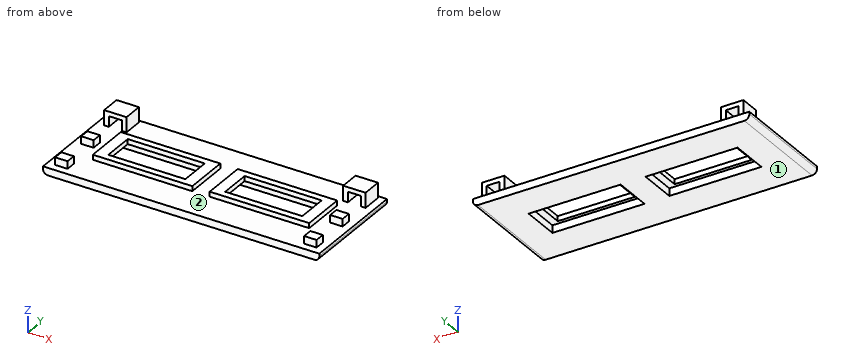
```python
from build123d import *

# Parameters (mm, degrees)
SKETCH1_W           = 111.1
SKETCH1_H           = 51.3
BOSS_EXTRUDE1_DEPTH = 3
SKETCH2_W           = 111.1
SKETCH2_H           = 51.3
SKETCH2_W_2         = 105.3
SKETCH2_H_2         = 45.3
BOSS_EXTRUDE2_DEPTH = 40.5
SKETCH10_W          = 126.244554882
SKETCH10_H          = 68.697179438
CUT_EXTRUDE2_DEPTH  = 53
SKETCH11_W          = 5
SKETCH11_H          = 4
BOSS_EXTRUDE7_DEPTH = 3
SKETCH12_W          = 9
SKETCH12_H          = 8
BOSS_EXTRUDE8_DEPTH = 6
SKETCH13_W          = 5.2
SKETCH13_H          = 4.2
CUT_EXTRUDE3_DEPTH  = 12
FILLET2_R           = 2
SKETCH5_W           = 37
SKETCH5_H           = 15.3
CUT_EXTRUDE5_DEPTH  = 3
SKETCH15_W          = 40
SKETCH15_H          = 18
SKETCH15_W_2        = 31
SKETCH15_H_2        = 12.5
BOSS_EXTRUDE9_DEPTH = 2


with BuildPart() as part:
    # Sketch1 → Boss-Extrude1 (new body)
    with BuildSketch(Plane(origin=(0, 0, 0), x_dir=(1, 0, 0), z_dir=(0, 1, 0))):
        Rectangle(SKETCH1_W, SKETCH1_H)
    extrude(amount=BOSS_EXTRUDE1_DEPTH)

    # Sketch2 → Boss-Extrude2 (add)
    with BuildSketch(Plane(origin=(0, 3, 0), x_dir=(1, 0, 0), z_dir=(0, 1, 0))):
        Rectangle(SKETCH2_W, SKETCH2_H)
        Rectangle(SKETCH2_W_2, SKETCH2_H_2, mode=Mode.SUBTRACT)
    extrude(amount=BOSS_EXTRUDE2_DEPTH)

    # Sketch10 → Cut-Extrude2 (cut)
    with BuildSketch(Plane.XY.offset(-22.65)):
        with Locations((0, 21.75)):
            Rectangle(SKETCH10_W, SKETCH10_H)
    extrude(amount=CUT_EXTRUDE2_DEPTH, mode=Mode.SUBTRACT)

    # Sketch11 → Boss-Extrude7 (add)
    with BuildSketch(Plane.XY.offset(-22.65)):
        with Locations((-50.05, 21.75)):
            Rectangle(SKETCH11_W, SKETCH11_H)
        with Locations((-50.05, 5)):
            Rectangle(SKETCH11_W, SKETCH11_H)
        with Locations((50.05, 5)):
            Rectangle(SKETCH11_W, SKETCH11_H)
        with Locations((50.05, 21.75)):
            Rectangle(SKETCH11_W, SKETCH11_H)
    extrude(amount=BOSS_EXTRUDE7_DEPTH)

    # Sketch12 → Boss-Extrude8 (add)
    with BuildSketch(Plane.XY.offset(-22.65)):
        with Locations((-48.05, 38.5)):
            Rectangle(SKETCH12_W, SKETCH12_H)
        with Locations((48.05, 38.5)):
            Rectangle(SKETCH12_W, SKETCH12_H)
    extrude(amount=BOSS_EXTRUDE8_DEPTH)

    # Sketch13 → Cut-Extrude3 (cut)
    with BuildSketch(Plane(origin=(0, 42.5, 0), x_dir=(1, 0, 0), z_dir=(0, 1, 0))):
        with Locations((-48.05, 20.55)):
            Rectangle(SKETCH13_W, SKETCH13_H)
        with Locations((48.05, 20.55)):
            Rectangle(SKETCH13_W, SKETCH13_H)
    extrude(amount=-CUT_EXTRUDE3_DEPTH, mode=Mode.SUBTRACT)

    # Fillet2
    fillet2_edges = [part.edges().sort_by_distance(p)[0] for p in [
        (-55.55, 21.75, -25.65),
        (55.55, 21.75, -25.65),
    ]]
    fillet(fillet2_edges, radius=FILLET2_R)

    # Sketch5 → Cut-Extrude5 (cut)
    with BuildSketch(Plane(origin=(0, 0, -25.65), x_dir=(-1, 0, 0), z_dir=(0, 0, -1))):
        with Locations((23.5, 21.75)):
            Rectangle(SKETCH5_W, SKETCH5_H)
        with Locations((-23.5, 21.75)):
            Rectangle(SKETCH5_W, SKETCH5_H)
    extrude(amount=-CUT_EXTRUDE5_DEPTH, mode=Mode.SUBTRACT)

    # Sketch15 → Boss-Extrude9 (add)
    # profile 1 of 2: a face of its own
    with BuildSketch(Plane.XY.offset(-22.65)):
        with Locations((23.5, 21.75)):
            Rectangle(SKETCH15_W, SKETCH15_H)
        with Locations((23.5, 21.75)):
            Rectangle(SKETCH15_W_2, SKETCH15_H_2, mode=Mode.SUBTRACT)
    # profile 2 of 2: a face of its own
    with BuildSketch(Plane.XY.offset(-22.65)):
        with Locations((-23.5, 21.75)):
            Rectangle(SKETCH15_W, SKETCH15_H)
        with Locations((-23.5, 21.75)):
            Rectangle(SKETCH15_W_2, SKETCH15_H_2, mode=Mode.SUBTRACT)
    extrude(amount=BOSS_EXTRUDE9_DEPTH)


solid = part.part
```
For this review, take the finished solid that the model builds, in its own axes (mm). Face numbers are marked on the shaded views. Coordinates: 2 decimals unless noted, no trailing zeros. Order: outer loops, then holes, each group sorted by start corner. A loop starts at its lowest first (then second) coordinate and runs counter-clockwise, first axis right, second up. Notation, with made-up numbers: (85, 27) - (93, 27) arc R26 cw to (93, 65) - close; hole circle Ø11 at (53.25, -39.75). An arc over 180 degrees is marked (long way). Answer as a JSON object with one key per item and string values. Group by question number.
1. The part is to be moulded in two halves that separate along X. For the marked faces 1 and 2, say which applies: pulls with the +X half, pulls with the -X half, needs draft (parallel to the pull), parting line crosses it, or undercut.
2. We need section A-A on x = -46.5. State the section outline as (y, z) points, then the cut area to 3 significant figures.
3. We need section B-B on y = 18. Give the number of separate pieces and of enclosed holes in the cut face, then the cut area to 3 significant figures.
4. We need section C-C on x = -0.5. State the section outline as (y, z) points.
5. For probe 1 along X at (y, z) = (38, -19.75); probe 2 along Y at (x, z) = (19, -21.5); probe 3 along Y at (x, z) = (41, -25), list the stretches that pass through material, from the lowest coordinate up.
6. Clearance check with flat-ended pins moving along their axes: P1, Ø1.5, axis at x = 50, z = -20.5, coming from the -Y side; P2, Ø1.5, axis at y = 22, z = -21.5, coming from the +X side; P3, Ø1.5, axis at y = 21, z = -20.5, coming from the -X side. State where each tip first meets the part, or that it passes through.
Final values:
{
 "1": {"face 1": "needs draft", "face 2": "undercut"},
 "2": {"outline": "(0, -25.65) - (43.5, -25.65) - (43.5, -22.65) - (0, -22.65) - close; (34.5, -18.45) - (42.5, -18.45) - (42.5, -16.65) - (34.5, -16.65) - close", "area": "145 mm²"},
 "3": {"separate pieces": "3", "enclosed holes": "0", "area": "146 mm²"},
 "4": {"outline": "(0, -25.65) - (43.5, -25.65) - (43.5, -22.65) - (0, -22.65) - close"},
 "5": {"probe 1": "-52.55 to -50.65, -45.45 to -43.55, 43.55 to 45.45, 50.65 to 52.55", "probe 2": "12.75 to 15.5, 28 to 30.75", "probe 3": "0 to 14.1, 29.4 to 43.5"},
 "6": {"P1": "y = 3", "P2": "x = 52.55", "P3": "x = -52.55"}
}
